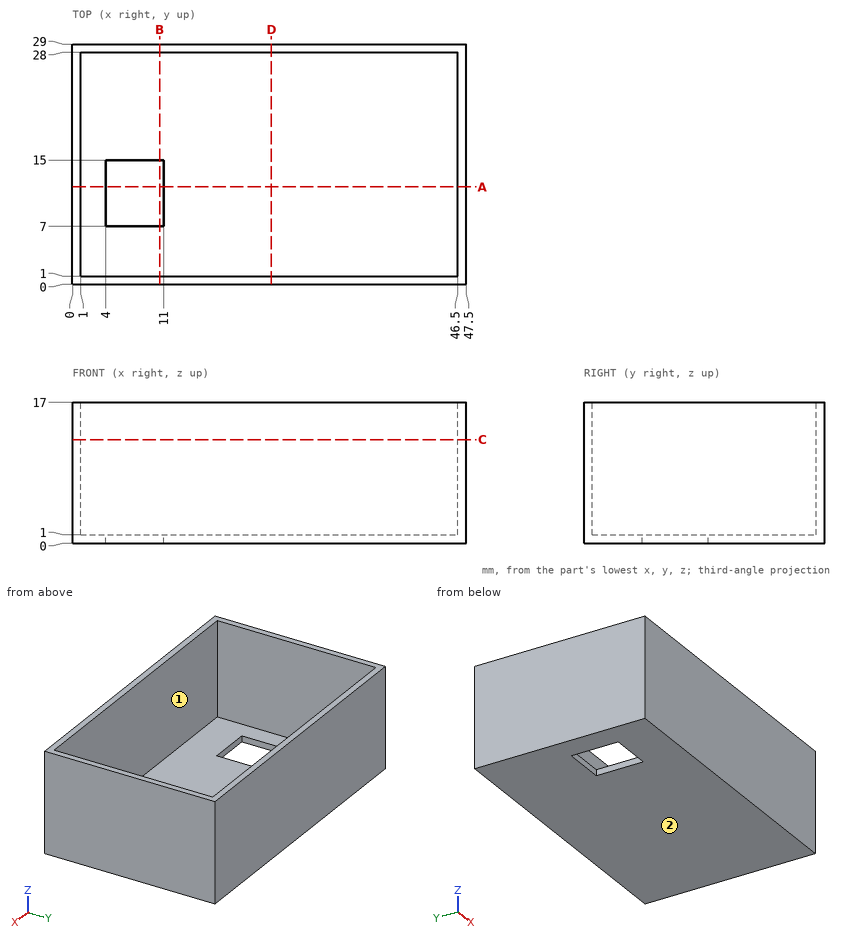
For this review, use the dimensioned drawing (mm, ordinates from the lowest corner) and the shaded views. A direction names the side the tool comes from. Give positions to 0.01 mm unless a question says otherwise; leave off trailing zeros. Loops run counter-clockwise (first coordinate to the right, second up) from the corner with the lowest first, then second, coordinate; pieces in that order, holes last. Notation, with made-up numbers: (65, 3.5) -> (118, 3.5) arc R24 ccw to (118, 36.5) -> close; hole circle Ø5 at (21.25, 11.25). An arc over 180 degrees is marked (long way). One line per question, with ' | ' between items. Start each with the question number.
(1) We need section B-B (x = 10.5). State the section outline as (y, z) points, and give its area (3 significant figures).
(2) For line 1 (X direction, y = 25.5, z = 9.5); line 2 (Y direction, x = 19, z = 15); line 3 (Y direction, x = 6.5, z = 0.75), list the stretches that pass through material, from the lowest coordinate up.
(3) Insertion check: P1, Ø4, axis at x = 42.5, y = 11.5, coming from the +Z side. The pin has a flat end and moves straight along its axis. Give the tip position at first contact, or say it passes through.
(4) We need section A-A (y = 11.75). State the section outline as (x, z) points.
(5) We need section D-D (x = 24). State the section outline as (y, z) points, and give its area (3 significant figures).
(6) For the marked faces 1 and 2, list the 3-axis set-ups (+Z, -Z, +X, -X, +Y, -Y) from which the entire face can be reached by the end or side of a thin tool; tool diameter is ignored.
(7) We need section C-C (z = 12.5). State the section outline as (x, y) points, and give its area (3 significant figures).
The answers:
1) outline: (0, 0) -> (7, 0) -> (7, 1) -> (1, 1) -> (1, 17) -> (0, 17) -> close; (15, 0) -> (29, 0) -> (29, 17) -> (28, 17) -> (28, 1) -> (15, 1) -> close | area: 53.0 mm^2
2) line 1: x = 0 to 1, 46.5 to 47.5 | line 2: y = 0 to 1, 28 to 29 | line 3: y = 0 to 7, 15 to 29
3) P1: stops at z = 1
4) outline: (0, 0) -> (4, 0) -> (4, 1) -> (1, 1) -> (1, 17) -> (0, 17) -> close; (11, 0) -> (47.5, 0) -> (47.5, 17) -> (46.5, 17) -> (46.5, 1) -> (11, 1) -> close
5) outline: (0, 0) -> (29, 0) -> (29, 17) -> (28, 17) -> (28, 1) -> (1, 1) -> (1, 17) -> (0, 17) -> close | area: 61.0 mm^2
6) face 1: +Z | face 2: -Z, +X, -X, +Y, -Y
7) outline: (0, 0) -> (47.5, 0) -> (47.5, 29) -> (0, 29) -> close; hole (1, 1) -> (46.5, 1) -> (46.5, 28) -> (1, 28) -> close | area: 149 mm^2
